from build123d import *

# Parameters (mm, degrees)
BOSS_EXTRUDE1_DEPTH     = 38.1
SKETCH2_R               = 9.8806
CUT_EXTRUDE1_DEPTH      = 128.791284914
CUT_EXTRUDE2_DEPTH      = 89.045446362
CUT_EXTRUDE2_DEPTH_BACK = 89.045446362
SKETCH3_R               = 3.175
SKETCH4_W               = 46.294
SKETCH4_H               = 2.54
CUT_EXTRUDE3_DEPTH      = 98.602206085


with BuildPart() as part:
    # Sketch1 → Boss-Extrude1 (new body)
    with BuildSketch(Plane(origin=(0, 0, 0), x_dir=(1, 0, 0), z_dir=(0, 1, 0))):
        with BuildLine():
            Line((-47.625, 76.2), (-47.625, 12.7))
            ThreePointArc((-47.625, 12.7), (-43.905256121, 3.719743879), (-34.925, 0))
            Line((-34.925, 0), (34.925, 0))
            ThreePointArc((34.925, 0), (43.905256121, 3.719743879), (47.625, 12.7))
            Line((47.625, 12.7), (47.625, 76.2))
            Line((47.625, 76.2), (26.797, 76.2))
            Line((26.797, 76.2), (26.797, 22.7))
            ThreePointArc((26.797, 22.7), (23.868067812, 15.628932188), (16.797, 12.7))
            Line((16.797, 12.7), (-16.797, 12.7))
            ThreePointArc((-16.797, 12.7), (-23.868067812, 15.628932188), (-26.797, 22.7))
            Line((-26.797, 22.7), (-26.797, 76.2))
            Line((-26.797, 76.2), (-47.625, 76.2))
        make_face()
    extrude(amount=BOSS_EXTRUDE1_DEPTH)

    # Sketch2 → Cut-Extrude1 (cut, through all)
    with BuildSketch(Plane(origin=(47.625, 0, 0), x_dir=(0, 0, -1), z_dir=(1, 0, 0))):
        with Locations((52.324, 19.05)):
            Circle(SKETCH2_R)
    extrude(amount=-CUT_EXTRUDE1_DEPTH, mode=Mode.SUBTRACT)

    # Sketch3 → Cut-Extrude2 (cut, two sides: drawn at the far end of the back side and taken through both)
    with BuildSketch(Plane(origin=(0, 0, -12.7), x_dir=(-1, 0, 0), z_dir=(0, 0, -1)).offset(-CUT_EXTRUDE2_DEPTH_BACK)):
        with Locations((-16.797, 19.05)):
            Circle(SKETCH3_R)
        with Locations((16.797, 19.05)):
            Circle(SKETCH3_R)
    extrude(amount=CUT_EXTRUDE2_DEPTH + CUT_EXTRUDE2_DEPTH_BACK, mode=Mode.SUBTRACT)

    # Sketch4 → Cut-Extrude3 (cut, through all)
    with BuildSketch(Plane.XZ):
        with Locations((0, -13.97)):
            Rectangle(SKETCH4_W, SKETCH4_H)
    extrude(amount=-CUT_EXTRUDE3_DEPTH, mode=Mode.SUBTRACT)


solid = part.part
Model file for the job. Use its own axes, mm. A direction names the side the tool comes from. Coordinates: 2 decimals unless noted, no trailing zeros. Order: outer loops, then holes, each group sorted by start corner. A loop starts at its lowest first (then second) coordinate and runs counter-clockwise, first axis right, second up. Notation, with made-up numbers: M 79.25,-3.5 L 130.25,-3.5 A16 ccw 130.25,24.5 Z; hole C -2,59.5 d8. An arc over 180 degrees is marked long. Return JSON: item names as keys, results as strings.
1. Flat gauge pin, fed straight in: pin 1 (11.5 mm diameter, centred on x = 0.5, y = 15, fed in from -Z). Where does the tip first touch, or does it go through?
Ans:
{"pin 1": "z = -12.7"}
2. Tool access for faces 1 (the face through (0, 19, 0)), 2 (the face through (26.797, 27, -44)): list every direction of +Z, -Z, +X, -X, +Y, -Y with a clear straight run to the whole face (end or side of a thin tool).
Ans:
{"face 1": "+Z, +X, -X, +Y, -Y", "face 2": "-Z, +Y, -Y"}
3. Saw through at C-C (x = 29.5). Give the cut face in (y, z), and give its area (3 significant figures).
Ans:
{"outline": "M 0,-76.2 L 38.1,-76.2 L 38.1,0 L 0,0 Z; hole C 19.05,-52.32 d19.76", "area": "2,600 mm^2"}
4. Drill centre lines: probe 1 along X at (y, z) = (3, -28.5) (3 decimals); probe 2 along X at (y, z) = (18.5, -7); probe 3 along X at (y, z) = (19, -5). Where is each one in solid material? Low to high.
Ans:
{"probe 1": "-47.625 to -26.797, 26.797 to 47.625", "probe 2": "-46.27 to -19.92, -13.67 to 13.67, 19.92 to 46.27", "probe 3": "-45.02 to -19.97, -13.62 to 13.62, 19.97 to 45.02"}
5. Saw through at D-D (y = 30.5). Give the cut face in (x, z) (3 decimals).
Ans:
{"outline": "M -47.625,-76.2 L -26.797,-76.2 L -26.797,-22.7 A10 cw -23.147,-14.975 L -23.147,-12.7 L 23.147,-12.7 L 23.147,-14.975 A10 cw 26.797,-22.7 L 26.797,-76.2 L 47.625,-76.2 L 47.625,-12.7 A12.7 ccw 34.925,0 L -34.925,0 A12.7 ccw -47.625,-12.7 Z"}
6. Saw through at B-B (y = 19.05). Give the number of separate pieces and of enclosed holes in the cut face, and give its area (3 significant figures).
Ans:
{"separate pieces": "5", "enclosed holes": "0", "area": "2,830 mm^2"}
7. Pull direction Y, two halves, no side cores. Call faces 3 (the face through (-44.003, 18.783, -3.819)), 4 (the face through (-1, 0, -5)), 5 (the face through (-16.11, 15.95, -6.26)): +Y half, -Y half, draft (parallel to the pull), parting line (faces both ways), or undercut.
Ans:
{"face 3": "draft", "face 4": "-Y half", "face 5": "undercut"}
8. Saw through at A-A (z = -29). Give the cut face in (x, y) (3 decimals), and give its area (3 significant figures).
Ans:
{"outline": "M -47.625,0 L -26.797,0 L -26.797,38.1 L -47.625,38.1 Z; M 26.797,0 L 47.625,0 L 47.625,38.1 L 26.797,38.1 Z", "area": "1,590 mm^2"}
